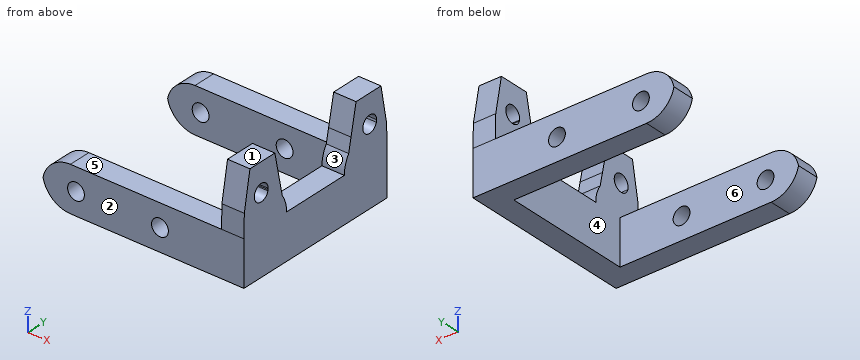
from build123d import *

# Parameters (mm, degrees)
F0_W        = 32
F0_H        = 4
F1_DEPTH    = 8
F3_DEPTH    = 4
F4_DEPTH    = 25
F5_R        = 1.5
F6_DEPTH    = 40
F7_T1_DEPTH = 29
F7_T3_DEPTH = 29


# Not quite as in the source:
# - a fillet or chamfer that OpenCascade refuses, or shapes differently, is made with other operations: its cross-section is extruded or revolved along the edge and cut away or added


with BuildPart() as f1:
    # F0 (on Top) → F1 (new body)
    with BuildSketch(Plane.XY):
        with Locations((-2, 13.5)):
            Rectangle(F0_W, F0_H)
        Polygon((14, 11.5), (14, -11.5), (14, -15.5), (18, -15.5), (18, 0), (18, 15.5), (14, 15.5), align=None)
        with Locations((-2, -13.5)):
            Rectangle(F0_W, F0_H)
    extrude(amount=F1_DEPTH)

    # F2 (on face) → F3 (join, through all)
    with BuildSketch(Plane.YZ.offset(18)):
        with BuildLine():
            Line((-15.4216540828, 12.0949916113), (-15.5, 8))
            Line((-15.5, 8), (-6.25, 8))
            ThreePointArc((-6.25, 8), (-6.4923756022, 9.6147401314), (-7.1981402517, 11.0871625858))
            ThreePointArc((-7.1981402517, 11.0871625858), (-8.5517740167, 12.4745223834), (-10.3026318448, 13.3061403509))
            ThreePointArc((-10.3026318448, 13.3061403509), (-11.75, 12.2), (-13.1973681552, 13.3061403509))
            ThreePointArc((-13.1973681552, 13.3061403509), (-14.3801744212, 12.8303397928), (-15.4216540828, 12.0949916113))
        make_face()
        with BuildLine():
            Line((6.25, 8), (11.75, 8))
            Line((11.75, 8), (15.5, 8))
            Line((15.5, 8), (15.4216540828, 12.0949916113))
            ThreePointArc((15.4216540828, 12.0949916113), (14.3801744212, 12.8303397928), (13.1973681552, 13.3061403509))
            ThreePointArc((13.1973681552, 13.3061403509), (11.75, 12.2), (10.3026318448, 13.3061403509))
            ThreePointArc((10.3026318448, 13.3061403509), (8.5517740167, 12.4745223834), (7.1981402517, 11.0871625858))
            ThreePointArc((7.1981402517, 11.0871625858), (6.4923756022, 9.6147401314), (6.25, 8))
        make_face()
        with BuildLine():
            Line((-14.1999293119, 18.7123082578), (-15.4216540828, 12.0949916113))
            ThreePointArc((-15.4216540828, 12.0949916113), (-14.3801744212, 12.8303397928), (-13.1973681552, 13.3061403509))
            ThreePointArc((-13.1973681552, 13.3061403509), (-11.9486803553, 15.1867838163), (-10.25, 13.7))
            ThreePointArc((-10.25, 13.7), (-10.2533520267, 13.5997760311), (-10.2633931253, 13.5))
            Line((-10.2633931253, 13.5), (-7.7054746686, 13.5))
            Line((-7.7054746686, 13.5), (-8.8014388457, 18.7123082578))
            Line((-8.8014388457, 18.7123082578), (-14.1999293119, 18.7123082578))
        make_face()
        with BuildLine():
            ThreePointArc((-10.3026318448, 13.3061403509), (-8.5517740167, 12.4745223834), (-7.1981402517, 11.0871625858))
            Line((-7.1981402517, 11.0871625858), (-7.7054746686, 13.5))
            Line((-7.7054746686, 13.5), (-10.2633931253, 13.5))
            ThreePointArc((-10.2633931253, 13.5), (-10.2798136989, 13.4024227159), (-10.3026318448, 13.3061403509))
        make_face()
        with BuildLine():
            ThreePointArc((13.1973681552, 13.3061403509), (14.3801744212, 12.8303397928), (15.4216540828, 12.0949916113))
            Line((15.4216540828, 12.0949916113), (14.1999293119, 18.7123082578))
            Line((14.1999293119, 18.7123082578), (8.8014388457, 18.7123082578))
            Line((8.8014388457, 18.7123082578), (7.7054746686, 13.5))
            Line((7.7054746686, 13.5), (10.2633931253, 13.5))
            ThreePointArc((10.2633931253, 13.5), (11.6497760311, 15.1966479733), (13.25, 13.7))
            ThreePointArc((13.25, 13.7), (13.2367838163, 13.5013196447), (13.1973681552, 13.3061403509))
        make_face()
        with BuildLine():
            Line((7.7054746686, 13.5), (7.1981402517, 11.0871625858))
            ThreePointArc((7.1981402517, 11.0871625858), (8.5517740167, 12.4745223834), (10.3026318448, 13.3061403509))
            ThreePointArc((10.3026318448, 13.3061403509), (10.2798136989, 13.4024227159), (10.2633931253, 13.5))
            Line((10.2633931253, 13.5), (7.7054746686, 13.5))
        make_face()
    extrude(amount=-F3_DEPTH)

    # F2 (on face) → F4 (cut)
    with BuildSketch(Plane.YZ.offset(18)):
        with BuildLine():
            ThreePointArc((10.2633931253, 13.5), (10.2798136989, 13.4024227159), (10.3026318448, 13.3061403509))
            ThreePointArc((10.3026318448, 13.3061403509), (11.0198534153, 13.4513196535), (11.75, 13.5))
            Line((11.75, 13.5), (10.2633931253, 13.5))
        make_face()
        with BuildLine():
            ThreePointArc((11.75, 13.5), (11.0198534153, 13.4513196535), (10.3026318448, 13.3061403509))
            ThreePointArc((10.3026318448, 13.3061403509), (11.75, 12.2), (13.1973681552, 13.3061403509))
            ThreePointArc((13.1973681552, 13.3061403509), (12.4801465847, 13.4513196535), (11.75, 13.5))
        make_face()
        with BuildLine():
            ThreePointArc((11.75, 13.5), (12.4801465847, 13.4513196535), (13.1973681552, 13.3061403509))
            ThreePointArc((13.1973681552, 13.3061403509), (13.2367838163, 13.5013196447), (13.25, 13.7))
            ThreePointArc((13.25, 13.7), (11.6497760311, 15.1966479733), (10.2633931253, 13.5))
            Line((10.2633931253, 13.5), (11.75, 13.5))
        make_face()
        with BuildLine():
            ThreePointArc((-11.75, 13.5), (-12.4801465847, 13.4513196535), (-13.1973681552, 13.3061403509))
            ThreePointArc((-13.1973681552, 13.3061403509), (-11.75, 12.2), (-10.3026318448, 13.3061403509))
            ThreePointArc((-10.3026318448, 13.3061403509), (-11.0198534153, 13.4513196535), (-11.75, 13.5))
        make_face()
        with BuildLine():
            ThreePointArc((-11.75, 13.5), (-11.0198534153, 13.4513196535), (-10.3026318448, 13.3061403509))
            ThreePointArc((-10.3026318448, 13.3061403509), (-10.2798136989, 13.4024227159), (-10.2633931253, 13.5))
            Line((-10.2633931253, 13.5), (-11.75, 13.5))
        make_face()
        with BuildLine():
            ThreePointArc((-10.25, 13.7), (-11.9486803553, 15.1867838163), (-13.1973681552, 13.3061403509))
            ThreePointArc((-13.1973681552, 13.3061403509), (-12.4801465847, 13.4513196535), (-11.75, 13.5))
            Line((-11.75, 13.5), (-10.2633931253, 13.5))
            ThreePointArc((-10.2633931253, 13.5), (-10.2533520267, 13.5997760311), (-10.25, 13.7))
        make_face()
    extrude(amount=-F4_DEPTH, mode=Mode.SUBTRACT)

    # F5 (on face) → F6 (cut)
    with BuildSketch(Plane.XZ.offset(15.5)):
        with Locations((-12, 4)):
            Circle(F5_R)
        with Locations((3, 4)):
            Circle(F5_R)
    extrude(amount=-F6_DEPTH, mode=Mode.SUBTRACT)

    # F7: fillet of radius 5 on 4 edges, made by hand

    # F7_s2 → F7_t1 (cut)
    with BuildSketch(Plane.XZ.offset(-1)):
        with BuildLine():
            ThreePointArc((-18, 3), (-16.5355339059, 6.5355339059), (-13, 8))
            Line((-13, 8), (-18, 8))
            Line((-18, 8), (-18, 3))
        make_face()
        with BuildLine():
            ThreePointArc((-13, 0), (-16.5355339059, 1.4644660941), (-18, 5))
            Line((-18, 5), (-18, 0))
            Line((-18, 0), (-13, 0))
        make_face()
    extrude(amount=F7_T1_DEPTH, mode=Mode.SUBTRACT)

    # F7_s4 → F7_t3 (cut)
    with BuildSketch(Plane.XZ.offset(-28)):
        with BuildLine():
            ThreePointArc((-18, 3), (-16.5355339059, 6.5355339059), (-13, 8))
            Line((-13, 8), (-18, 8))
            Line((-18, 8), (-18, 3))
        make_face()
        with BuildLine():
            ThreePointArc((-18, 5), (-16.5355339059, 1.4644660941), (-13, 0))
            Line((-13, 0), (-18, 0))
            Line((-18, 0), (-18, 5))
        make_face()
    extrude(amount=F7_T3_DEPTH, mode=Mode.SUBTRACT)


solid = f1.part
The model under review builds one solid part; all positions refer to its coordinate system, in mm. Face numbers are marked on the shaded views. A direction names the side the tool comes from. Coordinates: 2 decimals unless noted, no trailing zeros. Order: outer loops, then holes, each group sorted by start corner. A loop starts at its lowest first (then second) coordinate and runs counter-clockwise, first axis right, second up. Notation, with made-up numbers: (46.25, 42.5) -> (89.25, 42.5) arc R27 ccw to (89.25, 80.5) -> close; hole circle Ø4 at (-20.75, -19). An arc over 180 degrees is marked (long way). Answer in a Markdown table with one row per item.
(1) The part is to be moulded in two halves that separate along Y. For the marked faces 1, 2 and 3, say which applies: +Y half, -Y half, draft (parallel to the pull), parting line (faces both ways), or undercut.
Answers:
| item | result |
|---|---|
| face 1 | draft |
| face 2 | -Y half |
| face 3 | undercut |
(2) Wall thickness on line 1 along Y through (x, z) = (-6, 3.75); line 2 along Z through (x, y) = (-12, 14); line 3 along Z through (x, y) = (16.45, -11.75): over which ranges is each line inside the solid? List them lowest first.
Answers:
| item | result |
|---|---|
| line 1 | -15.5 to -11.5, 11.5 to 15.5 |
| line 2 | 0 to 2.5, 5.5 to 8 |
| line 3 | 0 to 12.2, 15.2 to 18.71 |
(3) Machinability: for the marked faces 4, 5 and 6, which of the approach directions +Z, -Z, +X, -X, +Y, -Y give a long, thin tool a straight path to every point of the face, cutting with its end or side? Answer none if there is none.
Answers:
| item | result |
|---|---|
| face 4 | +Z, -X |
| face 5 | +Z, -X, +Y, -Y |
| face 6 | +Z, -Z, -X |
(4) Consider section A-A (x = -12). Write out the cut boundary in (y, z), plus the area to 3 significant figures.
Answers:
| item | result |
|---|---|
| outline | (-15.5, 0) -> (-11.5, 0) -> (-11.5, 2.5) -> (-15.5, 2.5) -> close; (-15.5, 5.5) -> (-11.5, 5.5) -> (-11.5, 8) -> (-15.5, 8) -> close; (11.5, 0) -> (15.5, 0) -> (15.5, 2.5) -> (11.5, 2.5) -> close; (11.5, 5.5) -> (15.5, 5.5) -> (15.5, 8) -> (11.5, 8) -> close |
| area | 40.0 mm² |
(5) Consider section B-B (y = -12). Write out the cut boundary in (x, z).
Answers:
| item | result |
|---|---|
| outline | (-17.9, 4) arc R5 ccw to (-13, 0) -> (18, 0) -> (18, 12.22) -> (14, 12.22) -> (14, 8) -> (-13, 8) arc R5 ccw to start; (14, 15.18) -> (18, 15.18) -> (18, 18.71) -> (14, 18.71) -> close; hole circle Ø3 at (-12, 4); hole circle Ø3 at (3, 4) |
(6) Consider section C-C (x = -3). Write out the cut boundary in (y, z).
Answers:
| item | result |
|---|---|
| outline | (-15.5, 0) -> (-11.5, 0) -> (-11.5, 8) -> (-15.5, 8) -> close; (11.5, 0) -> (15.5, 0) -> (15.5, 8) -> (11.5, 8) -> close |
(7) Insertion check: pin 1 (4 mm diameter, centred on y = -11.75, z = 13.7, fed in from -X); pin 2 (6.5 mm diameter, centred on x = 3.5, z = 3, fed in from +Y); pin 3 (1.2 mm diameter, centred on x = 15, y = 2, fed in from +Z). Each pin has a flat end and moves straight along its axis. Give the tip position at first contact, or say it passes through.
Answers:
| item | result |
|---|---|
| pin 1 | x = 14 |
| pin 2 | y = 15.5 |
| pin 3 | z = 8 |
(8) Consider section D-D (z = 3.5). Write out the cut boundary in (x, y).
Answers:
| item | result |
|---|---|
| outline | (-17.77, -15.5) -> (-13.41, -15.5) -> (-13.41, -11.5) -> (-17.77, -11.5) -> close; (-17.77, 11.5) -> (-13.41, 11.5) -> (-13.41, 15.5) -> (-17.77, 15.5) -> close; (-10.59, -15.5) -> (1.59, -15.5) -> (1.59, -11.5) -> (-10.59, -11.5) -> close; (-10.59, 11.5) -> (1.59, 11.5) -> (1.59, 15.5) -> (-10.59, 15.5) -> close; (4.41, -15.5) -> (18, -15.5) -> (18, 15.5) -> (4.41, 15.5) -> (4.41, 11.5) -> (14, 11.5) -> (14, -11.5) -> (4.41, -11.5) -> close |
